```python
from build123d import *

# Parameters (mm, degrees)
F1_R     = 5
F3_DEPTH = 38
F0_R     = 15
F4_DEPTH = 65
F5_DEPTH = 65
F6_DEPTH = 65
F7_R     = 16


with BuildPart() as f2:
    # F0 (on Front) → F2 (revolve)
    with BuildSketch(Plane.XZ):
        Polygon((75, 23), (72.5, 23), (72.5, -17), (72.5, -38), (72.5, -52), (75, -52), align=None)
    revolve(axis=Axis((56, 0, -14.5), (0, 0, -1)))

    # F1 (on Top) → F3 (join)
    with BuildSketch(Plane.XY):
        Polygon((-22, -29.475761), (-22, 29.475761), (-76.065856, 0), align=None)
        with Locations((-44, 0)):
            Circle(F1_R, mode=Mode.SUBTRACT)
        Polygon((22, -53.463793), (22, 53.463793), (-22, 29.475761), (-22, -29.475761), align=None)
        with BuildLine():
            ThreePointArc((72, -4.031129), (39.5, 0), (72, 4.031129))
            Line((72, 4.031129), (72, 80.722921))
            Line((72, 80.722921), (22, 53.463793))
            Line((22, 53.463793), (22, -53.463793))
            Line((22, -53.463793), (72, -80.722921))
            Line((72, -80.722921), (72, -4.031129))
        make_face()
        with Locations((56, -56)):
            Circle(F1_R, mode=Mode.SUBTRACT)
        with Locations((56, 56)):
            Circle(F1_R, mode=Mode.SUBTRACT)
    extrude(amount=-F3_DEPTH)

    # F0 (on Front) → F4 (cut, symmetric)
    with BuildSketch(Plane.XZ):
        Circle(F0_R)
    extrude(amount=F4_DEPTH, both=True, mode=Mode.SUBTRACT)

    # F0 (on Front) → F5 (join, symmetric)
    with BuildSketch(Plane.XZ):
        with BuildLine():
            ThreePointArc((13.96424, -17), (19.889863, -9.401774), (22, 0))
            ThreePointArc((22, 0), (0, 22), (-22, 0))
            ThreePointArc((-22, 0), (-9.401774, -19.889863), (13.96424, -17))
        make_face()
        Circle(F0_R, mode=Mode.SUBTRACT)
    extrude(amount=F5_DEPTH, both=True)

    # F1 (on Top) → F6 (cut, symmetric)
    with BuildSketch(Plane.XY):
        with BuildLine():
            ThreePointArc((72, -4.031129), (72.374523, -2.03101), (72.5, 0))
            ThreePointArc((72.5, 0), (72.374523, 2.03101), (72, 4.031129))
            Line((72, 4.031129), (72, 0))
            Line((72, 0), (72, -4.031129))
        make_face()
    extrude(amount=F6_DEPTH, both=True, mode=Mode.SUBTRACT)

    # F7
    f7_edges = [f2.edges().sort_by_distance(p)[0] for p in [
        (-76.065856, 0, -19),
        (72, -80.722921, -19),
        (72, 80.722921, -19),
    ]]
    fillet(f7_edges, radius=F7_R)


solid = f2.part
```
Design review of the part built by this model. Coordinates are the model's own, in mm. A direction names the side the tool comes from. Give positions to 0.01 mm unless a question says otherwise; leave off trailing zeros. Write each loop counter-clockwise with the first axis right and the second up, starting at its lowest first coordinate (ties: lowest second). Pieces come first, ordered by that corner, then holes. Notation, with made-up numbers: (-37.75, 80.25) - (13.25, 80.25) arc R11 ccw to (13.25, 100.25) - close; hole circle Ø6 at (-29, -34.75). An arc over 180 degrees is marked (long way). Return JSON: item names as keys, results as strings. Group by question number.
(1) We need section C-C, the plane x = -43. Give the boundary of the cut face in (y, z).
(2) We need section D-D, the plane z = 18.5. Give the boundary of the cut face in (x, y), then the cut area to 3 significant figures.
(3) We need section B-B, the plane z = -6. Give the boundary of the cut face in (x, y).
(4) To check wall thickness, follow probe 1 along Y at (x, z) = (56, -18); probe 2 along X at (y, z) = (-51.5, -18); probe 3 along Y at (x, z) = (17.5, -32). State the ranges of each line that lie inside material, in increasing order.
(5) Mouldability with a two-part tool opening along Y and no side actions: class faces 5 (the cylindrical face through (64.367, 67.414, -19.266)), 6 (the cylindrical face through (39.516, -0.725, -15.025)), 7 (the flat face through (36, 1, 0)) as +Y half, -Y half, draft (parallel to the pull), parting line (faces both ways), or undercut.
(6) Insertion check: pin 1 (11.5 mm diameter, centred on y = 32, z = -12.5, fed in from +X); pin 2 (4 mm diameter, centred on y = 1.5, z = -5, fed in from -X); pin 3 (8 mm diameter, centred on x = 21, y = 20.5, fed in from +Z); pin 4 (13 mm diameter, centred on x = -4, z = 10.5, fed in from +Y). Each pin has a flat end and moves straight along its axis. Give the tip position at first contact, or say it passes through.
(7) Machinability: for faces 1 (the flat face through (14.4, -65, 5.2)), 2 (the flat face through (72, 32, -19)), 3 (the flat face through (72, -32, -19)), 4 (the cylindrical face through (73.55, 7.28, -13.98)), which of the approach directions +Z, -Z, +X, -X, +Y, -Y give a long, thin tool a straight path to every point of the face, cutting with its end or side? Answer none if there is none.
(8) We need section A-A, the plane y = 0. Give the boundary of the cut face in (x, z), then the cut area to 3 significant figures.
Reported:
{
 "1": {"outline": "(-18.03, -38) - (-4.9, -38) - (-4.9, 0) - (-18.03, 0) - close; (4.9, -38) - (18.03, -38) - (18.03, 0) - (4.9, 0) - close"},
 "2": {"outline": "(-11.91, -65) - (11.91, -65) - (11.91, 65) - (-11.91, 65) - close; circle Ø38 at (56, 0); hole circle Ø33 at (56, 0)", "area": "3,370 mm2"},
 "3": {"outline": "(-50.3, -14.05) - (-21.17, -29.93) - (-21.17, -65) - (-13.75, -65) - (-13.75, 65) - (-21.17, 65) - (-21.17, 29.93) - (-50.3, 14.05) arc R16 ccw to start; (13.75, -65) - (21.17, -65) - (21.17, -53.01) - (48.34, -67.82) arc R16 ccw to (72, -53.78) - (72, -10.25) arc R19 ccw to (72, 10.25) - (72, 53.78) arc R16 ccw to (48.34, 67.82) - (21.17, 53.01) - (21.17, 65) - (13.75, 65) - close; hole circle Ø10 at (-44, 0); hole circle Ø33 at (56, 0); hole circle Ø10 at (56, -56); hole circle Ø10 at (56, 56)"},
 "4": {"probe 1": "y = -69.78 to -61, -51 to -16.5, 16.5 to 51, 61 to 69.78", "probe 2": "x = -12.65 to 12.65, 18.4 to 53.82, 58.18 to 72", "probe 3": "y = -51.01 to 51.01"},
 "5": {"face 5": "+Y half", "face 6": "undercut", "face 7": "draft"},
 "6": {"pin 1": "stops at x = 72", "pin 2": "stops at x = -58.64", "pin 3": "stops at z = 13.96", "pin 4": "stops at y = 65"},
 "7": {"face 1": "+Z, -Z, -X, -Y", "face 2": "+Z, -Z, +X, +Y", "face 3": "+Z, -Z, +X, -Y", "face 4": "none"},
 "8": {"outline": "(-58.64, -38) - (-49, -38) - (-49, 0) - (-58.64, 0) - close; (-39, -38) - (37, -38) - (37, -52) - (39.5, -52) - (39.5, 23) - (37, 23) - (37, 0) - (22, 0) arc R22 ccw to (-22, 0) - (-39, 0) - close; (72.5, -52) - (75, -52) - (75, 23) - (72.5, 23) - close; hole circle Ø30 at (0, 0)", "area": "3,680 mm2"}
}
